Part model, mm, in its own coordinate system. A direction names the side the tool comes from. Give positions to 0.01 mm unless a question says otherwise; leave off trailing zeros. Order: outer loops, then holes, each group sorted by start corner. A loop starts at its lowest first (then second) coordinate and runs counter-clockwise, first axis right, second up. Notation, with made-up numbers: M 51,-9.75 L 91,-9.75 A31 ccw 91,28.25 Z; hole C 24.25,34 d6. An arc over 180 degrees is marked long. One line per question, with ' | ' between items.
```python
from build123d import *

# Parameters (mm, degrees)
SZKIC1_W                    = 74
SZKIC1_H                    = 9.7
DODANIE_WYCI_GNI_CIE1_DEPTH = 174
DODANIE_WYCI_GNI_CIE2_DEPTH = 2
SZKIC3_W                    = 25
SZKIC3_H                    = 0.2
DODANIE_WYCI_GNI_CIE3_DEPTH = 10
SZKIC4_W                    = 25
SZKIC4_H                    = 0.2
DODANIE_WYCI_GNI_CIE4_DEPTH = 10


with BuildPart() as part:
    # Szkic1 → Dodanie-wyciągnięcie1 (new body)
    with BuildSketch(Plane.XY):
        with Locations((37, -4.85)):
            Rectangle(SZKIC1_W, SZKIC1_H)
    extrude(amount=DODANIE_WYCI_GNI_CIE1_DEPTH)

    # Szkic2 → Dodanie-wyciągnięcie2 (add)
    with BuildSketch(Plane.XY.offset(174)):
        Polygon((3.5, 0), (3.5, -1), (33.5, -1), (33.5, 0), (18.5, 0), align=None)
        Polygon((40.5, 0), (40.5, -1), (70.5, -1), (70.5, 0), (55.5, 0), align=None)
    extrude(amount=DODANIE_WYCI_GNI_CIE2_DEPTH)

    # Szkic3 → Dodanie-wyciągnięcie3 (add)
    with BuildSketch(Plane.XY.offset(176)):
        with Locations((18.5, -0.5)):
            Rectangle(SZKIC3_W, SZKIC3_H)
    extrude(amount=DODANIE_WYCI_GNI_CIE3_DEPTH)

    # Szkic4 → Dodanie-wyciągnięcie4 (add)
    with BuildSketch(Plane.XY.offset(176)):
        with Locations((55.5, -0.5)):
            Rectangle(SZKIC4_W, SZKIC4_H)
    extrude(amount=DODANIE_WYCI_GNI_CIE4_DEPTH)


solid = part.part
```
1. Tool access for faces 1 (the flat face through (18, -0.6, 181)), 2 (the flat face through (74, -5, 86)), 3 (the flat face through (55, -0.4, 181)): list every direction of +Z, -Z, +X, -X, +Y, -Y with a clear straight run to the whole face (end or side of a thin tool).
Worked out:
face 1: +Z, +X, -X, -Y | face 2: +Z, -Z, +X, +Y, -Y | face 3: +Z, +X, -X, +Y
2. Probe L1, parallel to Z at x = 69.5, y = -2.75. List the from-to ranges inside material, lowest first. Write a range as from..to.
Worked out:
L1: z = 0..174
3. Slice it at C-C on x = 37.5. Give the cut face in (y, z).
Worked out:
outline: M -9.7,0 L 0,0 L 0,174 L -9.7,174 Z
4. Slice it at A-A on x = 62.5. Give the cut face in (y, z).
Worked out:
outline: M -9.7,0 L 0,0 L 0,176 L -0.4,176 L -0.4,186 L -0.6,186 L -0.6,176 L -1,176 L -1,174 L -9.7,174 Z
5. Slice it at B-B on y = -4.75. Give the cut face in (x, z).
Worked out:
outline: M 0,0 L 74,0 L 74,174 L 0,174 Z
6. Drop flat-ended pins along their axis: pin 1 (1.1 mm diameter, centred on y = -0.5, z = 175.5, fed in from -X); pin 2 (5 mm diameter, centred on x = 19.5, y = -4.5, fed in from +Z); pin 3 (8 mm diameter, centred on x = 16.5, z = 181, fed in from -Y). Give the stop position or say it passes through.
Worked out:
pin 1: stops at x = 3.5 | pin 2: stops at z = 174 | pin 3: stops at y = -0.6
